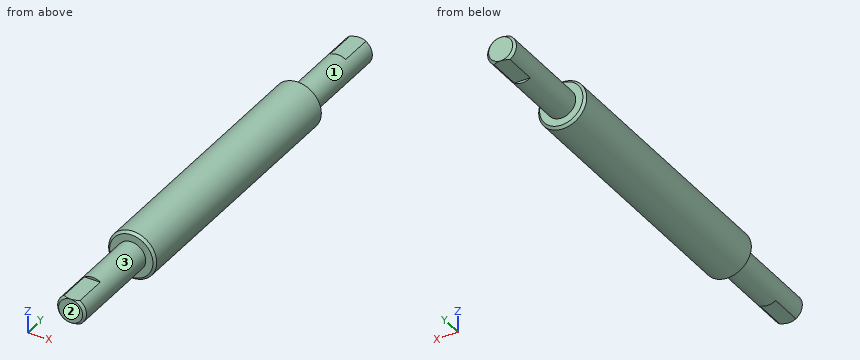
Autodesk Inventor part; units mm, degrees
ref_plane "YZ Plane" through (0, 0, 0) normal (1, 0, 0) x (0, 1, 0)
ref_plane "XZ Plane" through (0, 0, 0) normal (0, 1, 0) x (-1, 0, 0)
ref_plane "XY Plane" through (0, 0, 0) normal (0, 0, 1) x (1, 0, 0)
sketch "Sketch1" plane through (0, 0, 0) normal (0, 1, 0) x (-1, 0, 0)
  circle A0 centre (0, 0) radius 3
  dimension "d0" = 6
extrude "Extrusion1" add sketch "Sketch1" along normal blind 100
chamfer "Chamfer1" distance 0.5 angle 45 2 edges at (3, 100, 0) (3, 0, 0)
sketch "Sketch3" plane through (0, 100, 0) normal (0, 1, 0) x (1, 0, 0)
  circle A0 centre (0, 0) radius 3
  line L0 (-1.6583, -2.5) -> (1.6583, -2.5)
  dimension "d16" = 2.5
extrude "Extrusion3" cut sketch "Sketch3" against normal blind 7.5 contours L0 A0 picked at (-0.3442, -2.6056)
mirror "Mirror1" about plane through (0, 0, 0) normal (0, 0, 1) of "Extrusion3"
ref_plane "Work Plane3" through (0, 50, 0) normal (0, -1, 0) x (1, 0, 0)
mirror "Mirror2" about plane through (0, 50, 0) normal (0, -1, 0) of "Extrusion3", "Mirror1"
sketch "Sketch4" plane through (0, 50, 0) normal (0, -1, 0) x (1, 0, 0)
  circle A0 centre (0, 0) radius 5
  dimension "d20" = 10
extrude "Extrusion4" add sketch "Sketch4" along normal mid plane 58
chamfer "Chamfer3" distance 0.5 angle 45 2 edges at (-5, 21, 0) (-5, 79, 0)
thread "Thread3"
properties part number "Вал"
Check sheet for the modelled part. Datum: model origin and axes. Units: mm. Face numbers are marked on the shaded views. A direction names the side the tool comes from. Round coordinates to 2 decimals unless told otherwise and drop trailing zeros. Loops run counter-clockwise (first coordinate to the right, second up) from the corner with the lowest first, then second, coordinate; pieces in that order, holes last. Notation, with made-up numbers: (9, -17.75) - (15, -17.75) arc R20 ccw to (15, -0.75) - close; hole circle Ø9 at (-1, -24.75). An arc over 180 degrees is marked (long way). Answer as CSV lines item,"result". Start each with the question number.
Item 1: Set-up check for the marked faces 1, 2 and 3: record each of +Z, -Z, +X, -X, +Y, -Y from which the full face is reachable in a straight line by a thin tool's end or side.
Item 2: Section check B-B (y = 20). Record the boundary of the cut face in (x, z), and give its area (3 significant figures).
Item 3: Section check A-A (z = 0). Record the boundary of the cut face in (x, y).
Item 4: Section check C-C (y = 70). Record the boundary of the cut face in (x, z), and give its area (3 significant figures).
Item 5: Scan lines: line 1 (X direction, y = 72, z = 0.25); line 2 (Y direction, x = 3.75, z = -0.25); line 3 (Z direction, x = -4, y = 24.5). Record each from-to range of solid material in increasing order. Write a range as [from, to].
Item 6: Depth check by flat-ended pin: P1, Ø3.5, axis at x = -1, y = 5, coming from the -Z side; P2, Ø5, axis at x = -3.5, y = 24.5, coming from the -Z side; P3, Ø3, axis at x = -3, y = 28, coming from the -Z side. Enter the tip coordinate at first touch or a pass-through.
Report:
1,face 1,"+Y"
1,face 2,"+Z, -Z, +X, -X, -Y"
1,face 3,"-Y"
2,outline,"circle Ø6 at (0, 0)"
2,area,"28.3 mm2"
3,outline,"(-5, 21.5) - (-4.5, 21) - (-3, 21) - (-3, 0.5) - (-2.5, 0) - (2.5, 0) - (3, 0.5) - (3, 21) - (4.5, 21) - (5, 21.5) - (5, 78.5) - (4.5, 79) - (3, 79) - (3, 99.5) - (2.5, 100) - (-2.5, 100) - (-3, 99.5) - (-3, 79) - (-4.5, 79) - (-5, 78.5) - close"
4,outline,"circle Ø10 at (0, 0)"
4,area,"78.5 mm2"
5,line 1,"x = [-4.99, 4.99]"
5,line 2,"y = [21, 79]"
5,line 3,"z = [-3, 3]"
6,P1,"stops at z = -2.5"
6,P2,"stops at z = -4.9"
6,P3,"stops at z = -4.77"
